from build123d import *

# Parameters (mm, degrees)
F0_W     = 20
F0_H     = 20
F2_W     = 15
F2_H     = 15
F4_R     = 5
F5_DEPTH = 11
F6_R     = 2.75
F7_DEPTH = 10


with BuildPart() as f3:
    # F0 (on Top) → F3 section 0
    with BuildSketch(Plane.XY):
        Rectangle(F0_W, F0_H)
    # F2 (on offset) → F3 section 1
    with BuildSketch(Plane.XY.offset(-15)):
        Rectangle(F2_W, F2_H)
    loft()

    # F4 (on face) → F5 (cut)
    with BuildSketch(Plane(origin=(0, 0, -15), x_dir=(1, 0, 0), z_dir=(0, 0, -1))):
        with Locations((0, -0.431754)):
            Circle(F4_R)
    extrude(amount=-F5_DEPTH, mode=Mode.SUBTRACT)

    # F6 (on face) → F7 (cut)
    with BuildSketch(Plane(origin=(0, 0, -4), x_dir=(1, 0, 0), z_dir=(0, 0, -1))):
        with Locations((0, -0.431754)):
            Circle(F6_R)
    extrude(amount=-F7_DEPTH, mode=Mode.SUBTRACT)


solid = f3.part
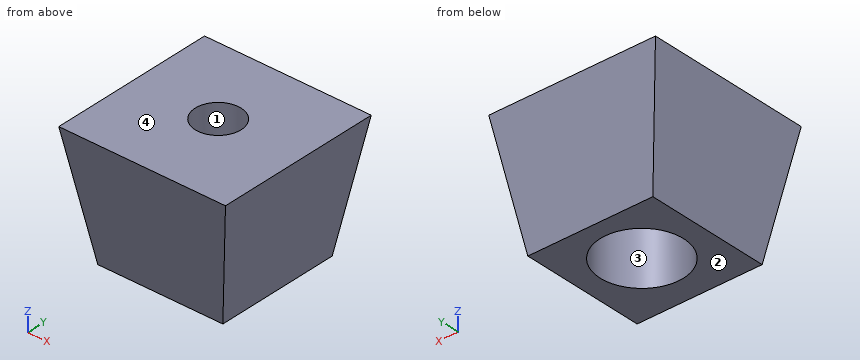
Verification items for the finished model (mm, model axes). Face numbers are marked on the shaded views. A direction names the side the tool comes from. Round coordinates to 2 decimals unless told otherwise and drop trailing zeros. Use a Markdown table: item, result. Add a question column.
1. Access from +Z, -Z, +X, -X, +Y, -Y to the whole of each face (thin tool, end or side, straight path). Record for the marked faces 3 and 4.
2. Gauge pin test, flat ends, axial feed: pin 1 (4 mm diameter, centred on x = 6, z = -8, fed in from +Y); pin 2 (2 mm diameter, centred on x = -7.5, z = -12.5, fed in from -Y); pin 3 (7 mm diameter, centred on x = 0, y = 0.43, fed in from -Z); pin 4 (1 mm diameter, centred on x = -1, y = -0.5, fed in from -Z). Record the tip position at first contact, or that the pin passes through.
3. Release check for a two-part mould opening along Y. For the marked faces 1 and 2 record: released by +Y, released by -Y, zero draft, split by the parting line, or undercut.
4. Thickness scan on probe 1 along Y at (x, z) = (0, -1.75); probe 2 along Z at (x, y) = (-0.25, -4); probe 3 along Y at (x, z) = (0, -10.5). Record the ranges inside material, lowest first. Write a range as [from, to].
Checks:
| question | item | result |
|---|---|---|
| 1 | face 3 | -Z |
| 1 | face 4 | +Z, +X, -X, +Y, -Y |
| 2 | pin 1 | stops at y = 9 |
| 2 | pin 2 | stops at y = -8.08 |
| 2 | pin 3 | stops at z = -4 |
| 2 | pin 4 | passes through |
| 3 | face 1 | undercut |
| 3 | face 2 | zero draft |
| 4 | probe 1 | y = [-9.71, -2.32], [3.18, 9.71] |
| 4 | probe 2 | z = [-4, 0] |
| 4 | probe 3 | y = [-8.25, -4.57], [5.43, 8.25] |
